```python
from build123d import *

# Parameters (mm, degrees)
EXTRU_MINCE1_DEPTH           = 2.3
CONG_1_R                     = 2.3
ESQUISSE2_W                  = 80
ESQUISSE2_H                  = 49.6
BOSS_EXTRU_1_DEPTH           = 2.3
R_P_TITION_START             = 77.7
R_P_TITION_LIN_AIRE1_DEPTH   = 4.6
R_P_TITION_START_2           = 37.7
R_P_TITION_LIN_AIRE1_2_DEPTH = 4.6
CONG_2_R                     = 2.3
BOSS_EXTRU_2_DEPTH           = 40
BOSS_EXTRU_2_DEPTH_BACK      = 25
BOSS_EXTRU_2_START           = -47.3
ESQUISSE5_W                  = 23.2
ESQUISSE5_H                  = 62
ENL_V_MAT_EXTRU_1_DEPTH      = 63.5
ESQUISSE6_OUTSIDE_W          = 110.274
ESQUISSE6_OUTSIDE_H          = 100.274
ENL_V_MAT_EXTRU_2_DEPTH      = 1.5


# Read off the part's stored shape, not the designer's step: Répétition linéaire1
with BuildPart() as part:
    # Esquisse1 → Extru.-Mince1 (new, symmetric)
    with BuildSketch(Plane.XY):
        Polygon((-4.3, -57), (-4.3, -47.3), (2.3, -47.3), (2.3, 2.3), (-8.9, 2.3), (-8.9, -12), (-4.3, -12), (-4.3, -2.3), (-2.3, -2.3), (-2.3, -42.7), (-8.9, -42.7), (-8.9, -57), align=None)
    extrude(amount=EXTRU_MINCE1_DEPTH, both=True)

    # Congé1
    cong_1_edges = [part.edges().sort_by_distance(p)[0] for p in [
        (-6.6, -57, -2.3),
        (-4.3, -52.15, -2.3),
        (-1, -47.3, -2.3),
        (2.3, -22.5, -2.3),
        (-3.3, 2.3, -2.3),
        (-8.9, -4.85, -2.3),
        (-6.6, -12, -2.3),
        (-4.3, -7.15, -2.3),
        (-3.3, -2.3, -2.3),
        (-2.3, -22.5, -2.3),
        (-5.6, -42.7, -2.3),
        (-8.9, -49.85, -2.3),
        (-5.6, -42.7, 2.3),
        (-2.3, -22.5, 2.3),
        (-3.3, -2.3, 2.3),
        (-4.3, -7.15, 2.3),
        (-6.6, -12, 2.3),
        (-8.9, -4.85, 2.3),
        (-3.3, 2.3, 2.3),
        (2.3, -22.5, 2.3),
        (-1, -47.3, 2.3),
        (-4.3, -52.15, 2.3),
        (-6.6, -57, 2.3),
        (-8.9, -49.85, 2.3),
    ]]
    fillet(cong_1_edges, radius=CONG_1_R - 0.0001)  # a hair under: the kernel refuses the full size

    # Esquisse2 → Boss.-Extru.1 (add)
    with BuildSketch(Plane(origin=(0, 0, 0), x_dir=(0, 0, -1), z_dir=(1, 0, 0))):
        with Locations((-40, -22.5)):
            Rectangle(ESQUISSE2_W, ESQUISSE2_H)
    extrude(amount=BOSS_EXTRU_1_DEPTH)

    # Répétition linéaire1 outline → Répétition linéaire1 (add)
    with BuildSketch(Plane.XY.offset(R_P_TITION_START)):
        Polygon((-8.9, 2.3), (-8.9, -12), (-4.3, -12), (-4.3, -2.3), (-2.3, -2.3), (-2.3, -42.7), (-8.9, -42.7), (-8.9, -57), (-4.3, -57), (-4.3, -47.3), (2.3, -47.3), (2.3, 2.3), align=None)
    extrude(amount=R_P_TITION_LIN_AIRE1_DEPTH)

    # R_p_tition lin_aire1 2 outline → R_p_tition lin_aire1 2 (add)
    with BuildSketch(Plane.XY.offset(R_P_TITION_START_2)):
        Polygon((0, 2.3), (-8.9, 2.3), (-8.9, -12), (-4.3, -12), (-4.3, -2.3), (-2.3, -2.3), (-2.3, -42.7), (-8.9, -42.7), (-8.9, -57), (-4.3, -57), (-4.3, -47.3), (0, -47.3), align=None)
    extrude(amount=R_P_TITION_LIN_AIRE1_2_DEPTH)

    # Congé2
    cong_2_edges = [part.edges().sort_by_distance(p)[0] for p in [
        (2.3, -22.5, 82.3),
        (-1, -47.3, 82.3),
        (-3.3, 2.3, 82.3),
        (-4.45, 2.3, 77.7),
        (-2.15, -47.3, 77.7),
        (-4.3, -52.15, 77.7),
        (-6.6, -57, 77.7),
        (-6.6, -12, 77.7),
        (-8.9, -4.85, 77.7),
        (-8.9, -49.85, 77.7),
        (-6.6, -57, 82.3),
        (-4.3, -52.15, 82.3),
        (-8.9, -4.85, 82.3),
        (-6.6, -12, 82.3),
        (-4.3, -7.15, 77.7),
        (-3.3, -2.3, 77.7),
        (-2.3, -22.5, 77.7),
        (-5.6, -42.7, 77.7),
        (-8.9, -49.85, 82.3),
        (-4.3, -7.15, 82.3),
        (-3.3, -2.3, 82.3),
        (-2.3, -22.5, 82.3),
        (-5.6, -42.7, 82.3),
        (-2.15, -47.3, 42.3),
        (-4.45, 2.3, 42.3),
        (-4.3, -7.15, 42.3),
        (-3.3, -2.3, 42.3),
        (-2.3, -22.5, 42.3),
        (-5.6, -42.7, 42.3),
        (-8.9, -49.85, 42.3),
        (-4.45, 2.3, 37.7),
        (-2.15, -47.3, 37.7),
        (-4.3, -52.15, 37.7),
        (-6.6, -57, 37.7),
        (-6.6, -12, 37.7),
        (-8.9, -4.85, 37.7),
        (-8.9, -49.85, 37.7),
        (-6.6, -57, 42.3),
        (-4.3, -52.15, 42.3),
        (-8.9, -4.85, 42.3),
        (-6.6, -12, 42.3),
        (-4.3, -7.15, 37.7),
        (-3.3, -2.3, 37.7),
        (-2.3, -22.5, 37.7),
        (-5.6, -42.7, 37.7),
    ]]
    fillet(cong_2_edges, radius=CONG_2_R - 0.0001)  # a hair under: the kernel refuses the full size

    # Esquisse4 → Boss.-Extru.2 (add, two sides: drawn at the far end of the back side and taken through both)
    with BuildSketch(Plane(origin=(0, 0, 0), x_dir=(1, 0, 0), z_dir=(0, 1, 0)).offset(BOSS_EXTRU_2_START - BOSS_EXTRU_2_DEPTH_BACK)):
        with BuildLine():
            Line((0, -72.5), (26, -72.5))
            ThreePointArc((26, -72.5), (26.707106781, -72.207106781), (27, -71.5))
            Line((27, -71.5), (27, -8.5))
            ThreePointArc((27, -8.5), (26.707106781, -7.792893219), (26, -7.5))
            Line((26, -7.5), (0, -7.5))
            Line((0, -7.5), (0, -72.5))
        make_face()
    extrude(amount=BOSS_EXTRU_2_DEPTH + BOSS_EXTRU_2_DEPTH_BACK)

    # Esquisse5 → Enlèv. mat.-Extru.1 (cut)
    with BuildSketch(Plane(origin=(0, -7.3, 0), x_dir=(1, 0, 0), z_dir=(0, 1, 0))):
        with Locations((13.9, -40)):
            Rectangle(ESQUISSE5_W, ESQUISSE5_H)
    extrude(amount=-ENL_V_MAT_EXTRU_1_DEPTH, mode=Mode.SUBTRACT)

    # Esquisse6 outside → Enlèv. mat.-Extru.2 (cut)
    with BuildSketch(Plane(origin=(27, 0, 0), x_dir=(0, 0, -1), z_dir=(1, 0, 0))):
        with Locations((-40, -35)):
            Rectangle(ESQUISSE6_OUTSIDE_W, ESQUISSE6_OUTSIDE_H)
        with BuildLine():
            Line((-66.708611763, -8.204239779), (-51.291388237, -18.999495909))
            ThreePointArc((-51.291388237, -18.999495909), (-49.927035053, -19.672320442), (-48.423506056, -19.903735688))
            Line((-48.423506056, -19.903735688), (-31.576493944, -19.903735688))
            ThreePointArc((-31.576493944, -19.903735688), (-30.072964947, -19.672320442), (-28.708611763, -18.999495909))
            Line((-28.708611763, -18.999495909), (-13.291388237, -8.204239779))
            ThreePointArc((-13.291388237, -8.204239779), (-11.927035053, -7.531415246), (-10.423506056, -7.3))
            Line((-10.423506056, -7.3), (-7.5, -7.3))
            Line((-7.5, -7.3), (-7.5, -72.3))
            Line((-7.5, -72.3), (-72.5, -72.3))
            Line((-72.5, -72.3), (-72.5, -7.3))
            Line((-72.5, -7.3), (-69.576493944, -7.3))
            ThreePointArc((-69.576493944, -7.3), (-68.072964947, -7.531415246), (-66.708611763, -8.204239779))
        make_face(mode=Mode.SUBTRACT)
    extrude(amount=-ENL_V_MAT_EXTRU_2_DEPTH, mode=Mode.SUBTRACT)


solid = part.part
```
Part model, mm, in its own coordinate system. A direction names the side the tool comes from. Round coordinates to 2 decimals unless told otherwise and drop trailing zeros. Loops run counter-clockwise (first coordinate to the right, second up) from the corner with the lowest first, then second, coordinate; pieces in that order, holes last.
Item 1: 3-axis set-ups, long thin cutter, end or side, ignore diameter. For faces 4 (the face through (-1.61, -22.81, 38.36)), 5 (the face through (-6.57, -56.57, 78.66)), 6 (the face through (-8.24, -4.95, 78.39)): which of +Z, -Z, +X, -X, +Y, -Y reach the whole face in a straight line?
Item 2: Cut at B-B, the plane x = 11. Give the cut face in (y, z), then the cut area to 3 significant figures.
Item 3: Cut at A-A, the plane y = -52. State how many separate pieces and enclosed holes the cut face has, then the cut area to 3 significant figures.
Item 4: Drill centre lines: line 1 (Z direction, x = 8, y = -18.5); line 2 (X direction, y = -28, z = 32); line 3 (Z direction, x = -7, y = -55). Where is each one in solid material? Low to high.
Item 5: Mould opens along Y. For faces 1 (the face through (13, -72.3, 40)), 2 (the face through (-3.254, -1.298, 38.102)), 3 (the face through (-8.24, -4.95, -1.61)) say: +Y half, -Y half, draft (parallel to the pull), parting line (faces both ways), or undercut.
Item 6: Cut at D-D, the plane z = 54.5. Give the cut face in (x, y).
Item 7: Drop flat-ended pins along their axis: P1, Ø3, axis at y = -22, z = 27, coming from the -X side; P2, Ø7, axis at x = 14, z = 40.5, coming from the +Y side; P3, Ø2, axis at x = -2.5, y = -23, coming from the -Z side. Give the stop position or say it passes through.
A:
1. face 4: none
1. face 5: +X, -X, -Y
1. face 6: -X, +Y, -Y
2. outline: (-72.3, 7.5) - (-7.3, 7.5) - (-7.3, 9) - (-70.8, 9) - (-70.8, 71) - (-7.3, 71) - (-7.3, 72.5) - (-72.3, 72.5) - close
2. area: 288 mm2
3. separate pieces: 4
3. enclosed holes: 1
3. area: 366 mm2
4. line 1: z = 7.5 to 9, 71 to 72.5
4. line 2: x = 0 to 2.3, 25.5 to 27
4. line 3: z = -2.26 to 2.26, 37.74 to 42.26, 77.74 to 82.26
5. face 1: -Y half
5. face 2: undercut
5. face 3: draft
6. outline: (0, -72.3) - (27, -72.3) - (27, -16.75) - (25.5, -16.75) - (25.5, -70.8) - (2.3, -70.8) - (2.3, 2.3) - (0, 2.3) - close
7. P1: stops at x = 0
7. P2: stops at y = -70.8
7. P3: stops at z = -1.74
